Source: CAD feature listing. Evaluate the final solid. Frame: model axes, mm. A direction names the side the tool comes from. Give positions to 0.01 mm unless a question says otherwise; leave off trailing zeros. Write each loop counter-clockwise with the first axis right and the second up, starting at its lowest first coordinate (ties: lowest second). Pieces come first, ordered by that corner, then holes. Notation, with made-up numbers: (51, 75.25) -> (106, 75.25) arc R12 ccw to (106, 79.25) -> close; hole circle Ø10 at (88.25, -12.5). An arc over 180 degrees is marked (long way). Use one line per item in the form item = value. Start each with the question number.
(1) Cut plane D-D, the plane z = -19.5. Output: boundary loops of the cut face in (x, y), and give its area (3 significant figures).
(2) Set-up query: faces 5 (the face through (-24.486, 14.875, -28.486)), 6 (the face through (15.5, -17, -5)), 7 (the face through (20, 15.5, -1)), 8 (the face through (-19.556, 24.287, -3.248)). Return all of +Z, -Z, +X, -X, +Y, -Y with unobstructed straight access to the full face (end or side cutting, diameter ignored); none if empty.
(3) Cut plane A-A, the plane x = 0. Output: boundary loops of the cut face in (y, z), and give its area (3 significant figures).
(4) Cut plane C-C, the plane x = -16.5. Output: boundary loops of the cut face in (y, z).
(5) Material intervals for line 1 along X through (y, z) = (19, -1); line 2 along Y through (x, z) = (20, -1.3); line 3 along X through (y, z) = (-3.5, -12), sorted ascending. Write a range as from..to.
(6) Draft query along X for faces 1 (the face through (20.195, -17.513, -1.819)), 2 (the face through (25.5, 6, -13)), 3 (the face through (-25.5, 6, -13)), 4 (the face through (-24.486, 11.787, -23.235)). Return one class per face: pulls with the +X half, pulls with the -X half, needs draft (parallel to the pull), parting line crosses it, or undercut.
(7) First-contact query: P1, Ø1.2, axis at x = -20, z = -9, coming from the -Y side; P2, Ø2.5, axis at y = 15.98, z = -29.5, coming from the -X side; P3, Ø1, axis at x = -21, z = -1.5, coming from the -Y side. Flat tips, straight axial feed; report the tip coordinate or a pass-through.
(8) Cut plane B-B, the plane y = -2. Output: boundary loops of the cut face in (x, z).
from build123d import *

# Parameters (mm, degrees)
SKETCH_W        = 47
SKETCH_H        = 50
SKETCH_R        = 10
SKETCH_R_2      = 1.5
PAD_DEPTH       = 2
SKETCH001_R     = 1.5
PAD001_DEPTH    = 2
SKETCH002_R     = 1.5
PAD002_DEPTH    = 8
SKETCH004_R     = 1.5
POCKET_DEPTH    = 8
PAD003_DEPTH    = 8
SKETCH005_R     = 1.5
POCKET001_DEPTH = 4
SKETCH006_R     = 1.5
SKETCH006_R_2   = 3.5
PAD004_DEPTH    = 2
SKETCH007_R     = 1.5
PAD005_DEPTH    = 8
SKETCH008_R     = 1.5
POCKET002_DEPTH = 8
PAD006_DEPTH    = 8
SKETCH010_R     = 1.5
POCKET003_DEPTH = 4
FILLET_R        = 3


with BuildPart() as body:
    # Sketch → Pad (new body)
    with BuildSketch(Plane.XY):
        Rectangle(SKETCH_W, SKETCH_H)
        Circle(SKETCH_R, mode=Mode.SUBTRACT)
        with Locations((-20, -19)):
            Circle(SKETCH_R_2, mode=Mode.SUBTRACT)
        with Locations((20, -19)):
            Circle(SKETCH_R_2, mode=Mode.SUBTRACT)
        with Locations((-20, 19)):
            Circle(SKETCH_R_2, mode=Mode.SUBTRACT)
        with Locations((20, 19)):
            Circle(SKETCH_R_2, mode=Mode.SUBTRACT)
    extrude(amount=PAD_DEPTH)

    # Sketch001 (on Face2 of Pad) → Pad001 (join)
    with BuildSketch(Plane.YZ.offset(23.5)):
        with BuildLine():
            Line((-25, 2), (25, 2))
            Line((25, -8), (25, 2))
            Line((22.505468, -27.843823), (25, -8))
            ThreePointArc((1.953944, -32.406741), (13.581707, -36.214738), (22.505468, -27.843823))
            Line((-13, -12.372281), (1.953944, -32.406741))
            ThreePointArc((-18.5, -9.5), (-16.620185, -12.602418), (-13, -12.372281))
            Line((-18.5, -8), (-18.5, -9.5))
            ThreePointArc((-18.5, -8), (-20.847064, -4.279548), (-25, -2.829168))
            Line((-25, 2), (-25, -2.829168))
        make_face()
        with Locations((-15, -9.5)):
            Circle(SKETCH001_R, mode=Mode.SUBTRACT)
        with Locations((15.980762, -19.5)):
            Circle(SKETCH001_R, mode=Mode.SUBTRACT)
        with Locations((5.980762, -19.5)):
            Circle(SKETCH001_R, mode=Mode.SUBTRACT)
        with Locations((10.980762, -24.5)):
            Circle(SKETCH001_R, mode=Mode.SUBTRACT)
        with Locations((15.980762, -29.5)):
            Circle(SKETCH001_R, mode=Mode.SUBTRACT)
        with Locations((5.980762, -29.5)):
            Circle(SKETCH001_R, mode=Mode.SUBTRACT)
    extrude(amount=PAD001_DEPTH)

    # Sketch002 (on Face9 of Pad001) → Pad002 (join)
    with BuildSketch(Plane(origin=(23.5, 0, 0), x_dir=(0, -1, 0), z_dir=(-1, 0, 0))):
        with BuildLine():
            Line((18.5, -8), (18.5, -9.5))
            ThreePointArc((11.5, -9.5), (15, -13), (18.5, -9.5))
            Line((11.5, -9.5), (11.5, 0))
            Line((25, 0), (11.5, 0))
            Line((25, 0), (25, -2.829168))
            ThreePointArc((25, -2.829168), (20.847064, -4.279548), (18.5, -8))
        make_face()
        with Locations((15, -9.5)):
            Circle(SKETCH002_R, mode=Mode.SUBTRACT)
    extrude(amount=PAD002_DEPTH)

    # Sketch004 (on Face35 of Pad002) → Pocket (cut)
    with BuildSketch(Plane.XY):
        with Locations((20, -19)):
            Circle(SKETCH004_R)
    extrude(amount=-POCKET_DEPTH, mode=Mode.SUBTRACT)

    # Sketch003 (on Face9 of Pad002) → Pad003 (join)
    with BuildSketch(Plane(origin=(23.5, 0, 0), x_dir=(0, -1, 0), z_dir=(-1, 0, 0))):
        with BuildLine():
            Line((-25, 0), (-15.5, 0))
            Line((-15.5, 0), (-15.5, -2))
            ThreePointArc((-17.5, -4), (-16.085786, -3.414214), (-15.5, -2))
            Line((-17.5, -4), (-22.5, -4))
            ThreePointArc((-25, -1.5), (-24.267767, -3.267767), (-22.5, -4))
            Line((-25, 0), (-25, -1.5))
        make_face()
    extrude(amount=PAD003_DEPTH)

    # Sketch005 (on Face41 of Pad003) → Pocket001 (cut)
    with BuildSketch(Plane.XY):
        with Locations((20, 19)):
            Circle(SKETCH005_R)
    extrude(amount=-POCKET001_DEPTH, mode=Mode.SUBTRACT)

    # Sketch006 (on Face2 of Pocket001) → Pad004 (join)
    with BuildSketch(Plane(origin=(-23.5, 0, 0), x_dir=(0, -1, 0), z_dir=(-1, 0, 0))):
        with BuildLine():
            Line((25, 2), (-25, 2))
            Line((-25, 2), (-25, -8))
            Line((-25, -8), (-22.505468, -27.843823))
            ThreePointArc((-22.505468, -27.843823), (-13.581707, -36.214738), (-1.953944, -32.406741))
            Line((-1.953944, -32.406741), (13, -12.372281))
            ThreePointArc((13, -12.372281), (16.620185, -12.602418), (18.5, -9.5))
            Line((18.5, -9.5), (18.5, -8))
            ThreePointArc((25, -2.829168), (20.847064, -4.279548), (18.5, -8))
            Line((25, -2.829168), (25, 2))
        make_face()
        with Locations((15, -9.5)):
            Circle(SKETCH006_R, mode=Mode.SUBTRACT)
        with Locations((-10.980762, -24.5)):
            Circle(SKETCH006_R_2, mode=Mode.SUBTRACT)
    extrude(amount=PAD004_DEPTH)

    # Sketch007 (on Face9 of Pad004) → Pad005 (join)
    with BuildSketch(Plane.YZ.offset(-23.5)):
        with BuildLine():
            Line((-11.5, 0), (-25, 0))
            Line((-25, 0), (-25, -2.829168))
            ThreePointArc((-18.5, -8), (-20.847064, -4.279548), (-25, -2.829168))
            Line((-18.5, -8), (-18.5, -9.5))
            ThreePointArc((-18.5, -9.5), (-15, -13), (-11.5, -9.5))
            Line((-11.5, 0), (-11.5, -9.5))
        make_face()
        with Locations((-15, -9.5)):
            Circle(SKETCH007_R, mode=Mode.SUBTRACT)
    extrude(amount=PAD005_DEPTH)

    # Sketch008 (on Face62 of Pad005) → Pocket002 (cut)
    with BuildSketch(Plane.XY):
        with Locations((-20, -19)):
            Circle(SKETCH008_R)
    extrude(amount=-POCKET002_DEPTH, mode=Mode.SUBTRACT)

    # Sketch009 (on Face9 of Pocket002) → Pad006 (join)
    with BuildSketch(Plane.YZ.offset(-23.5)):
        with BuildLine():
            Line((25, 0), (15.5, 0))
            Line((15.5, 0), (15.5, -2))
            ThreePointArc((15.5, -2), (16.085786, -3.414214), (17.5, -4))
            Line((17.5, -4), (22.5, -4))
            ThreePointArc((22.5, -4), (24.267767, -3.267767), (25, -1.5))
            Line((25, -1.5), (25, 0))
        make_face()
    extrude(amount=PAD006_DEPTH)

    # Sketch010 (on Face67 of Pad006) → Pocket003 (cut)
    with BuildSketch(Plane.XY):
        with Locations((-20, 19)):
            Circle(SKETCH010_R)
    extrude(amount=-POCKET003_DEPTH, mode=Mode.SUBTRACT)

    # Fillet
    fillet_edges = [body.edges().sort_by_distance(p)[0] for p in [
        (-19.5, -25, -2.829168),
        (-24.5, -25, -2.829168),
        (19.5, -25, -2.829168),
        (24.5, -25, -2.829168),
    ]]
    fillet(fillet_edges, radius=FILLET_R)


with BuildPart() as part_mirroring:
    # Part__Mirroring: instance of Body
    add(body.part.mirror(Plane(origin=(0, 0, 0), x_dir=(0, -1, 0), z_dir=(1, 0, 0))))


solid = part_mirroring.part
Geometry says:
q1.outline = (-25.5, -7.68) -> (-23.5, -7.68) -> (-23.5, 4.48) -> (-25.5, 4.48) -> close; (-25.5, 7.48) -> (-23.5, 7.48) -> (-23.5, 14.48) -> (-25.5, 14.48) -> close; (-25.5, 17.48) -> (-23.5, 17.48) -> (-23.5, 23.55) -> (-25.5, 23.55) -> close; (23.5, -7.68) -> (25.5, -7.68) -> (25.5, 23.55) -> (23.5, 23.55) -> close
q1.area = 113 mm^2
q2.face_5 = -X
q2.face_6 = -Z, +Y, -Y
q2.face_7 = -Z
q2.face_8 = -Z, +Y
q3.outline = (-25, 0) -> (-10, 0) -> (-10, 2) -> (-25, 2) -> close; (10, 0) -> (25, 0) -> (25, 2) -> (10, 2) -> close
q3.area = 60.0 mm^2
q4.outline = (-25, -0.31) arc R3 ccw to (-22.93, -3.16) arc R6.67 cw to (-18.5, -8) -> (-18.5, -9.5) arc R3.5 ccw to (-11.5, -9.5) -> (-11.5, 0) -> (15.5, 0) -> (15.5, -2) arc R2 ccw to (17.5, -4) -> (22.5, -4) arc R2.5 ccw to (25, -1.5) -> (25, 2) -> (-25, 2) -> close; hole circle Ø3 at (-15, -9.5)
q5.line_1 = -25.5..-21.5, -18.5..-15.5, 15.5..18.5, 21.5..25.5
q5.line_2 = -24.83..-20.5, -17.5..-11.5, 15.5..17.5, 20.5..25
q5.line_3 = -25.5..-23.5, 23.5..25.5
q6.face_1 = undercut
q6.face_2 = pulls with the +X half
q6.face_3 = pulls with the -X half
q6.face_4 = needs draft
q7.P1 = -18.5
q7.P2 = 23.5
q7.P3 = -24.92
q8.outline = (-25.5, -27.11) -> (-23.5, -27.11) -> (-23.5, 0) -> (-9.8, 0) -> (-9.8, 2) -> (-25.5, 2) -> close; (9.8, 0) -> (23.5, 0) -> (23.5, -27.11) -> (25.5, -27.11) -> (25.5, 2) -> (9.8, 2) -> close
